The listing builds one solid part. Answer for the finished solid, in the listing's coordinates (mm). A direction names the side the tool comes from. Coordinates: 2 decimals unless noted, no trailing zeros. Order: outer loops, then holes, each group sorted by start corner. A loop starts at its lowest first (then second) coordinate and runs counter-clockwise, first axis right, second up. Notation, with made-up numbers: (-8, 25) -> (44, 25) arc R22 cw to (44, 35) -> close; hole circle Ø7 at (-27, 85). An arc over 180 degrees is marked (long way). Write each question's results on one line, items separated by ' | '. Start each with the question number.
(1) Given pin 1 (0.5 mm diameter, centred on x = 40.5, z = -15, fed in from +Y); pin 2 (17 mm diameter, centred on x = 74.5, z = -20, fed in from -Y); pin 3 (10 mm diameter, centred on y = 5.5, z = -35, fed in from +X); pin 4 (1.2 mm diameter, centred on y = 11.5, z = -20, fed in from -X), each flat-ended and moving along its own axis, determine where each tip first touches the part or whether it passes through.
(2) A tool of negligible diameter and unlimited length cuts with its end or side. For faces 1 (the face through (11.5, 10, -36)), 2 (the face through (96, 16, -20)), 3 (the face through (11, 3.75, -20)), 4 (the face through (83.354, 1.014, -14.355)), from which of +Z, -Z, +X, -X, +Y, -Y can it reach the whole face along a straight path? Write none if from no direction.
(3) Determine the mould class of faces 5 (the face through (17.5, 10, -20)), 6 (the face through (40.165, 8.563, -24.192)), 7 (the face through (39, 19, -2)) for opening direction Y: +Y half, -Y half, draft (parallel to the pull), parting line (faces both ways), or undercut.
(4) Straight lines are drawn through the part: L1, parallel to Z at x = 40.5, y = 6.25 (3 decimals); L2, parallel to Z at x = 40.5, y = 10 (3 decimals); L3, parallel to Z at x = 74.5, y = 1.05. For each, find the intervals that lie inside material, in ascending order.
(5) The part is cut by section C-C, the plane y = 18.75. Give the vertices of the cut face in (x, z).
(6) The part is cut by section B-B, the plane x = 37. Give the vertices of the cut face in (y, z).
(7) The part is cut by section A-A, the plane y = 8. Give the vertices of the cut face in (x, z) (3 decimals).
```python
from build123d import *

# Parameters (mm, degrees)
BOSS_EXTRUDE1_DEPTH     = 20
SKETCH2_R               = 0.875
SKETCH2_W               = 41
SKETCH2_H               = 21
CUT_EXTRUDE2_DEPTH      = 7
SKETCH2_7_W             = 41
SKETCH2_7_H             = 10
SKETCH2_7_H_2           = 5.5
CUT_EXTRUDE3_DEPTH      = 18
SKETCH2_8_R             = 0.875
CUT_EXTRUDE4_DEPTH      = 16
SKETCH5_R               = 10.5
CUT_EXTRUDE5_DEPTH      = 16
SKETCH6_R               = 0.875
SKETCH6_W               = 23
SKETCH6_H               = 12.5
CUT_EXTRUDE6_DEPTH      = 17.5
FILLET1_R               = 5
SKETCH7_W               = 6
SKETCH7_H               = 5
SKETCH7_H_2             = 2.5
CUT_EXTRUDE7_DEPTH      = 4
CUT_EXTRUDE8_DEPTH      = 107.73448365
CUT_EXTRUDE8_DEPTH_BACK = 107.73448365
SKETCH8_W               = 6
SKETCH8_H               = 12.5


with BuildPart() as part:
    # Sketch1 → Boss-Extrude1 (new body)
    with BuildSketch(Plane(origin=(0, 0, 0), x_dir=(1, 0, 0), z_dir=(0, 1, 0))):
        with BuildLine():
            Line((0, 40), (0, 0))
            Line((0, 0), (80, 0))
            ThreePointArc((80, 0), (100, 20), (80, 40))
            Line((80, 40), (0, 40))
        make_face()
    extrude(amount=BOSS_EXTRUDE1_DEPTH)

    # Sketch2 → Cut-Extrude2 (cut)
    with BuildSketch(Plane(origin=(0, 20, 0), x_dir=(1, 0, 0), z_dir=(0, 1, 0))):
        with BuildLine():
            Line((30, 36), (30, 4))
            Line((30, 4), (80, 4))
            ThreePointArc((80, 4), (96, 20), (80, 36))
            Line((80, 36), (30, 36))
        make_face()
        with Locations(Location((40.5, 25, 0), (0, 0, 270))):
            Circle(SKETCH2_R, mode=Mode.SUBTRACT)
        with Locations(Location((40.5, 15, 0), (0, 0, 270))):
            Circle(SKETCH2_R, mode=Mode.SUBTRACT)
        with Locations(Location((88.5, 25, 0), (0, 0, 270))):
            Circle(SKETCH2_R, mode=Mode.SUBTRACT)
        with Locations(Location((88.5, 15, 0), (0, 0, 270))):
            Circle(SKETCH2_R, mode=Mode.SUBTRACT)
        with Locations((64.5, 20)):
            Rectangle(SKETCH2_W, SKETCH2_H, mode=Mode.SUBTRACT)
    extrude(amount=-CUT_EXTRUDE2_DEPTH, mode=Mode.SUBTRACT)

    # Sketch2<7> → Cut-Extrude3 (cut)
    with BuildSketch(Plane(origin=(0, 20, 0), x_dir=(1, 0, 0), z_dir=(0, 1, 0))):
        with Locations((64.5, 20)):
            Rectangle(SKETCH2_7_W, SKETCH2_7_H)
        with Locations((64.5, 12.25)):
            Rectangle(SKETCH2_7_W, SKETCH2_7_H_2)
        with Locations((64.5, 27.75)):
            Rectangle(SKETCH2_7_W, SKETCH2_7_H_2)
    extrude(amount=-CUT_EXTRUDE3_DEPTH, mode=Mode.SUBTRACT)

    # Sketch2<8> → Cut-Extrude4 (cut)
    with BuildSketch(Plane(origin=(0, 20, 0), x_dir=(1, 0, 0), z_dir=(0, 1, 0))):
        with Locations(Location((40.5, 25, 0), (0, 0, 270))):
            Circle(SKETCH2_8_R)
        with Locations(Location((40.5, 15, 0), (0, 0, 270))):
            Circle(SKETCH2_8_R)
        with Locations(Location((88.5, 25, 0), (0, 0, 270))):
            Circle(SKETCH2_8_R)
        with Locations(Location((88.5, 15, 0), (0, 0, 270))):
            Circle(SKETCH2_8_R)
    extrude(amount=-CUT_EXTRUDE4_DEPTH, mode=Mode.SUBTRACT)

    # Sketch5 → Cut-Extrude5 (cut)
    with BuildSketch(Plane(origin=(0, 2, 0), x_dir=(1, 0, 0), z_dir=(0, 1, 0))):
        with Locations(Location((74.5, 20, 0), (0, 0, 270))):
            Circle(SKETCH5_R)
    extrude(amount=-CUT_EXTRUDE5_DEPTH, mode=Mode.SUBTRACT)

    # Sketch6 → Cut-Extrude6 (cut)
    with BuildSketch(Plane.ZY):
        with Locations((-6.2, 10)):
            Circle(SKETCH6_R)
        with Locations((-33.8, 10)):
            Circle(SKETCH6_R)
        with Locations((-20, 10)):
            Rectangle(SKETCH6_W, SKETCH6_H)
    extrude(amount=-CUT_EXTRUDE6_DEPTH, mode=Mode.SUBTRACT)

    # Fillet1
    # the kernel refuses this fillet: 5 mm, written as the material it takes off along each edge
    with BuildSketch(Plane(origin=(80, 20, -40), x_dir=(0, -1, 0), z_dir=(-1, 0, 0))) as fillet1_piece_1:
        with BuildLine():
            CenterArc((FILLET1_R, FILLET1_R), FILLET1_R, 180, 90)
            Line((0, FILLET1_R), (0, 0))
            Line((0, 0), (FILLET1_R, 0))
        make_face()
    extrude(amount=92.5, mode=Mode.SUBTRACT)
    with BuildSketch(Plane(origin=(-12.5, 20, 0), x_dir=(0, 0, -1), z_dir=(1, 0, 0))) as fillet1_piece_2:
        with BuildLine():
            CenterArc((FILLET1_R, -FILLET1_R), FILLET1_R, 90, 90)
            Line((0, -FILLET1_R), (0, 0))
            Line((0, 0), (FILLET1_R, 0))
        make_face()
    extrude(amount=92.5, mode=Mode.SUBTRACT)
    with BuildSketch(Plane(origin=(80, 20, -20), x_dir=(0, 0, 1), z_dir=(-1, 0, 0))) as fillet1_piece_3:
        with BuildLine():
            CenterArc((20 - FILLET1_R, -FILLET1_R), FILLET1_R, 0, 90)
            Line((20 - FILLET1_R, 0), (20, 0))
            Line((20, 0), (20, -FILLET1_R))
        make_face()
    revolve(axis=Axis((80, 20, -20), (0, 1, 0)), revolution_arc=180, mode=Mode.SUBTRACT)

    # Sketch7 → Cut-Extrude7 (cut)
    with BuildSketch(Plane(origin=(0, 13, 0), x_dir=(1, 0, 0), z_dir=(0, 1, 0))):
        Polygon((85, 17.5), (85, 20), (85, 22.5), (44, 22.5), (44, 17.5), align=None)
        with Locations((41, 20)):
            Rectangle(SKETCH7_W, SKETCH7_H)
        with Locations((88, 18.75)):
            Rectangle(SKETCH7_W, SKETCH7_H_2)
        with Locations((88, 21.25)):
            Rectangle(SKETCH7_W, SKETCH7_H_2)
    extrude(amount=-CUT_EXTRUDE7_DEPTH, mode=Mode.SUBTRACT)

    # Sketch8 → Cut-Extrude8 (cut, two sides: drawn at the far end of the back side and taken through both)
    with BuildSketch(Plane(origin=(0, 0, -8.5), x_dir=(-1, 0, 0), z_dir=(0, 0, -1)).offset(-CUT_EXTRUDE8_DEPTH_BACK)):
        with Locations((-14.5, 10)):
            Rectangle(SKETCH8_W, SKETCH8_H)
    extrude(amount=CUT_EXTRUDE8_DEPTH + CUT_EXTRUDE8_DEPTH_BACK, mode=Mode.SUBTRACT)


solid = part.part
```
Established:
1) pin 1: stops at y = 4 | pin 2: passes through | pin 3: stops at x = 97.32 | pin 4: stops at x = 17.5
2) face 1: +Z, -Z | face 2: +Y | face 3: none | face 4: +Y, -Y
3) face 5: undercut | face 6: draft | face 7: +Y half
4) L1: z = -40 to -25.875, -24.125 to -15.875, -14.125 to 0 | L2: z = -40 to -25.875, -24.125 to -22.5, -17.5 to -15.875, -14.125 to 0 | L3: z = -40 to -30.5, -9.5 to 0
5) outline: (0, -38.31) -> (80, -38.31) arc R18.31 ccw to (80, -1.69) -> (0, -1.69) -> close; hole (30, -36) -> (80, -36) arc R16 ccw to (80, -4) -> (30, -4) -> close
6) outline: (0, -40) -> (15, -40) arc R5 ccw to (19.9, -36) -> (13, -36) -> (13, -4) -> (19.9, -4) arc R5 ccw to (15, 0) -> (0, 0) -> close
7) outline: (0, -40) -> (11.5, -40) -> (11.5, -31.5) -> (0, -31.5) -> close; (0, -8.5) -> (11.5, -8.5) -> (11.5, 0) -> (0, 0) -> close; (17.5, -40) -> (80, -40) arc R20 ccw to (80, 0) -> (17.5, 0) -> close; hole circle Ø1.75 at (40.5, -25); hole circle Ø1.75 at (40.5, -15); hole (44, -30.5) -> (85, -30.5) -> (85, -9.5) -> (44, -9.5) -> close; hole circle Ø1.75 at (88.5, -25); hole circle Ø1.75 at (88.5, -15)
